Print and shaded views of the part. All mm, measured from the part's lowest x, y and z. Round coordinates to 2 decimals unless told otherwise and drop trailing zeros. Write each loop counter-clockwise with the first axis right and the second up, starting at its lowest first coordinate (ties: lowest second). Pieces come first, ordered by that corner, then holes. Notation, with made-up numbers: (83, 70) - (119, 70) arc R9 cw to (119, 81) - close; hole circle Ø7 at (45.5, -10.5). An arc over 180 degrees is marked (long way). One line per item, written item: value.
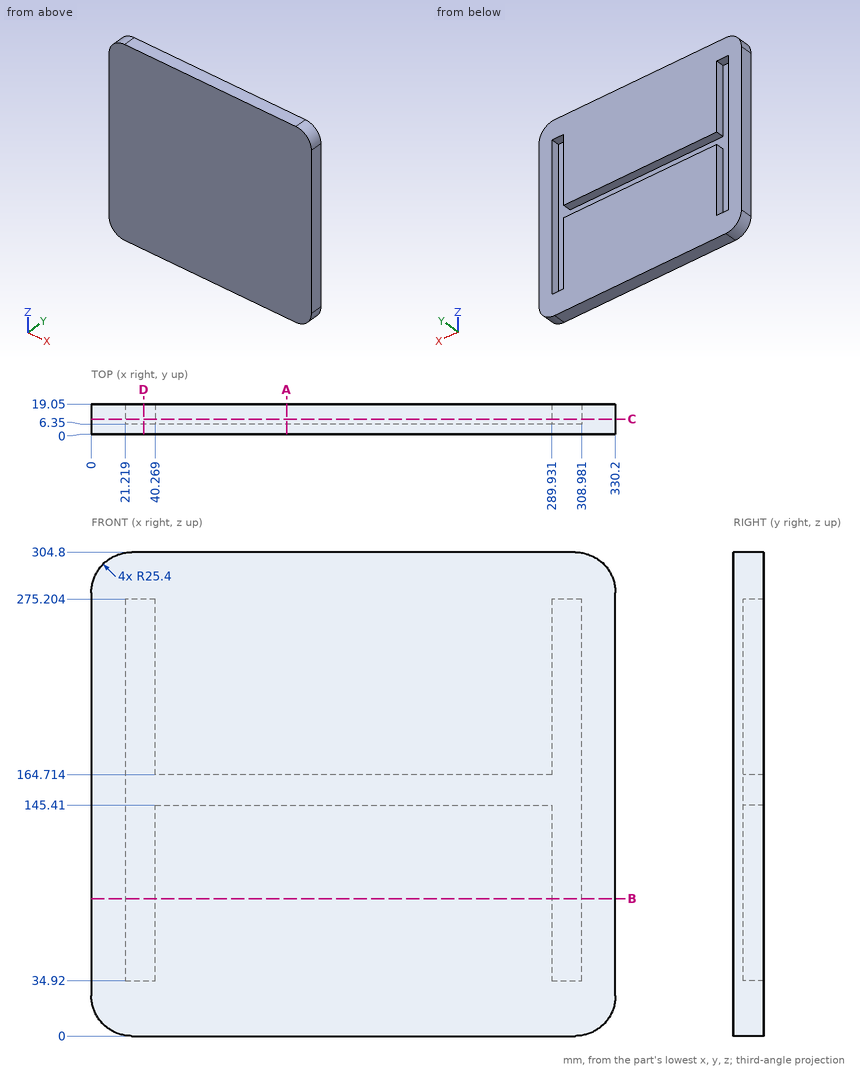
1. Band-saw the part on B-B on z = 86.5. Write the cut outline in (x, y).
Report:
outline: (0, 0) - (330.2, 0) - (330.2, 19.05) - (308.98, 19.05) - (308.98, 6.35) - (289.93, 6.35) - (289.93, 19.05) - (40.27, 19.05) - (40.27, 6.35) - (21.22, 6.35) - (21.22, 19.05) - (0, 19.05) - close
2. Band-saw the part on A-A on x = 123. Write the cut outline in (y, z).
Report:
outline: (0, 0) - (19.05, 0) - (19.05, 145.41) - (6.35, 145.41) - (6.35, 164.71) - (19.05, 164.71) - (19.05, 304.8) - (0, 304.8) - close
3. Band-saw the part on D-D on x = 33. Write the cut outline in (y, z).
Report:
outline: (0, 0) - (19.05, 0) - (19.05, 34.92) - (6.35, 34.92) - (6.35, 275.2) - (19.05, 275.2) - (19.05, 304.8) - (0, 304.8) - close
4. Wall check: probe 1 along X at (y, z) = (6.75, 264); probe 2 along X at (y, z) = (15.5, 154); probe 3 along Z at (x, y) = (196, 6.5). Give the ranges that are in metal, low to high. Write a range as [from, to].
Report:
probe 1: [0, 21.22], [40.27, 289.93], [308.98, 330.2]
probe 2: [0, 21.22], [308.98, 330.2]
probe 3: [0, 145.41], [164.71, 304.8]
5. Band-saw the part on C-C on y = 9.5. Write the cut outline in (x, z).
Report:
outline: (0, 25.4) arc R25.4 ccw to (25.4, 0) - (304.8, 0) arc R25.4 ccw to (330.2, 25.4) - (330.2, 279.4) arc R25.4 ccw to (304.8, 304.8) - (25.4, 304.8) arc R25.4 ccw to (0, 279.4) - close; hole (21.22, 34.92) - (40.27, 34.92) - (40.27, 145.41) - (289.93, 145.41) - (289.93, 34.92) - (308.98, 34.92) - (308.98, 275.2) - (289.93, 275.2) - (289.93, 164.71) - (40.27, 164.71) - (40.27, 275.2) - (21.22, 275.2) - close
